from build123d import *

# Parameters (mm, degrees)
SKETCH1_W                    = 55.5
SKETCH1_H                    = 76.5
BOSS_EXTRUDE1_DEPTH          = 4
BOSS_EXTRUDE2_DEPTH          = 3
F_4_0_4_DIAMETER_HOLE1_D     = 4
F_4_0_4_DIAMETER_HOLE1_DEPTH = 7


with BuildPart() as part:
    # Sketch1 → Boss-Extrude1 (new body)
    with BuildSketch(Plane(origin=(0, 0, 0), x_dir=(1, 0, 0), z_dir=(0, 1, 0))):
        with Locations((6.260396975, -11.980623819)):
            Rectangle(SKETCH1_W, SKETCH1_H)
    extrude(amount=BOSS_EXTRUDE1_DEPTH)

    # Sketch2 → Boss-Extrude2 (add)
    with BuildSketch(Plane(origin=(0, 4, 0), x_dir=(1, 0, 0), z_dir=(0, 1, 0))):
        Polygon((-21.489603025, 26.269376181), (-21.489603025, -50.230623819), (34.010396975, -50.230623819), (34.010396975, 26.269376181), (22.010396975, 26.269376181), (22.010396975, 19.269376181), (30.010396975, 19.269376181), (30.010396975, -33.230623819), (12.010396975, -33.230623819), (12.010396975, -45.230623819), (-15.489603025, -45.230623819), (-15.489603025, 20.269376181), (-7.489603025, 20.269376181), (-7.489603025, 22.269376181), (15.510396975, 22.269376181), (15.510396975, 26.269376181), align=None)
    extrude(amount=BOSS_EXTRUDE2_DEPTH)

    # Ø4.0 (4) Diameter Hole1
    with Locations(Plane(origin=(0, 7, 0), x_dir=(1, 0, 0), z_dir=(0, 1, 0))):
        with Locations((30.010396975, 22.269376181), (30.010396975, -46.230623819), (-17.489603025, -46.230623819), (-17.489603025, 22.269376181)):
            Hole(F_4_0_4_DIAMETER_HOLE1_D / 2, depth=F_4_0_4_DIAMETER_HOLE1_DEPTH)


solid = part.part
The listing builds one solid part. Answer for the finished solid, in the listing's coordinates (mm). A direction names the side the tool comes from. Round coordinates to 2 decimals unless told otherwise and drop trailing zeros. Write each loop counter-clockwise with the first axis right and the second up, starting at its lowest first coordinate (ties: lowest second). Pieces come first, ordered by that corner, then holes. Notation, with made-up numbers: (19.25, 18.25) - (44.25, 18.25) arc R13 ccw to (44.25, 26.25) - close; hole circle Ø8 at (76, 12). An arc over 180 degrees is marked (long way). Use one line per item in the form item = value. Start each with the question number.
Item 1: A tool of negligible diameter and unlimited length cuts with its end or side. For faces 1 (the flat face through (-15.49, 5, 13)), 2 (the cylindrical face through (-15.902, 3.451, -21.052)), from which of +Z, -Z, +X, -X, +Y, -Y can it reach the whole face along a straight path? Write none if from no direction.
Item 2: A flat-ended cylindrical pin translates along its axis: pin 1 Ø13.5 at (x, z) = (10, -0.5) entering from +Y. Find the tip coordinate at first contact, or state that the pin passes through.
Item 3: Find the intervals of material crossed by line 1 (Z direction, x = -5, y = 5.25); line 2 (X direction, y = 5.5, z = 2); line 3 (Z direction, x = 25, y = 6), in increasing order. Write a range as [from, to].
Item 4: A cutting plane is placed at D-D (x = 18.5). Write down the section's boundary in (y, z).
Item 5: A cutting plane is placed at A-A (z = 12). Write down the section's boundary in (x, y), plus the area to 3 significant figures.
Item 6: A cutting plane is placed at C-C (y = 5.5). Write down the section's boundary in (x, z), plus the area to 3 significant figures.
Item 7: Determine the mould class of faces 3 (the flat face through (12.01, 5, 39)), 4 (the flat face through (-7.49, 5, -21)), 5 (the flat face through (22.01, 5, -23)), 6 (the flat face through (6, 3, 50.231)) for opening direction Z: +Z half, -Z half, draft (parallel to the pull), parting line (faces both ways), or undercut.
Item 8: A cutting plane is placed at B-B (x = -0.5). Write down the section's boundary in (y, z).
The answers:
q1.face_1 = +Y
q1.face_2 = +Y, -Y
q2.pin_1 = 4
q3.line_1 = [-26.27, -22.27], [45.23, 50.23]
q3.line_2 = [-21.49, -15.49], [30.01, 34.01]
q3.line_3 = [-26.27, -19.27], [33.23, 50.23]
q4.outline = (0, -26.27) - (4, -26.27) - (4, 33.23) - (7, 33.23) - (7, 50.23) - (0, 50.23) - close
q5.outline = (-21.49, 0) - (34.01, 0) - (34.01, 7) - (30.01, 7) - (30.01, 4) - (-15.49, 4) - (-15.49, 7) - (-21.49, 7) - close
q5.area = 252 mm^2
q6.outline = (-21.49, -26.27) - (15.51, -26.27) - (15.51, -22.27) - (-7.49, -22.27) - (-7.49, -20.27) - (-15.49, -20.27) - (-15.49, 45.23) - (12.01, 45.23) - (12.01, 33.23) - (30.01, 33.23) - (30.01, -19.27) - (22.01, -19.27) - (22.01, -26.27) - (34.01, -26.27) - (34.01, 50.23) - (-21.49, 50.23) - close; hole circle Ø4 at (-17.49, -22.27); hole circle Ø4 at (-17.49, 46.23); hole circle Ø4 at (30.01, -22.27); hole circle Ø4 at (30.01, 46.23)
q6.area = 1,350 mm^2
q7.face_3 = undercut
q7.face_4 = undercut
q7.face_5 = draft
q7.face_6 = +Z half
q8.outline = (0, -26.27) - (7, -26.27) - (7, -22.27) - (4, -22.27) - (4, 45.23) - (7, 45.23) - (7, 50.23) - (0, 50.23) - close
